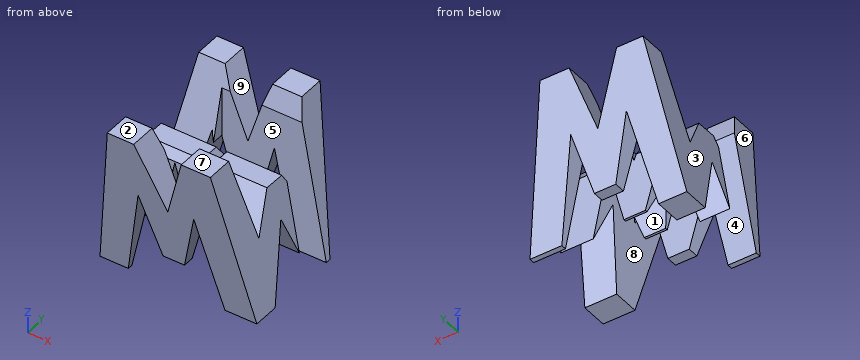
from build123d import *

# Parameters (mm, degrees)
F0_W      = 38.1
F0_H      = 38.1
F1_DEPTH  = 38.1
F6_DEPTH  = 38.1
F8_DEPTH  = 38.1
F9_W      = 25.4
F9_H      = 7.62
F10_DEPTH = 38.1


with BuildPart() as f1:
    # F0 (on Front) → F1 (new body)
    with BuildSketch(Plane.XZ):
        with Locations((19.05, 19.05)):
            Rectangle(F0_W, F0_H)
    extrude(amount=F1_DEPTH)

    # F4 (on face) → F6 (cut)
    with BuildSketch(Plane.YZ.offset(38.1)):
        Polygon((-6.35, 38.1), (-31.75, 38.1), (-26.67, 17.005277), (-21.59, 25.867645), (-16.51, 25.753345), (-11.43, 17.005277), align=None)
        Polygon((-31.75, 0), (-38.1, 38.1), (-38.1, 0), align=None)
        Polygon((0, 0), (0, 38.1), (-6.35, 0), align=None)
        Polygon((-19.05, 17.005277), (-25.4, 0), (-12.7, 0), align=None)
    extrude(amount=-F6_DEPTH, mode=Mode.SUBTRACT)

    # F7 (on offset) → F8 (cut)
    with BuildSketch(Plane.XZ.offset(38.1)):
        Polygon((0, 38.1), (0, 0), (6.205763, 38.1), align=None)
        Polygon((11.968254, 23.367919), (6.870665, 0), (30.363908, 0), (25.482736, 23.367919), (21.498529, 8.313587), (16.292483, 8.313587), align=None)
        Polygon((31.250443, 38.1), (38.1, 0), (38.1, 38.1), align=None)
        Polygon((24.158144, 38.1), (12.633159, 38.1), (19.05, 22.168303), align=None)
    extrude(amount=-F8_DEPTH, mode=Mode.SUBTRACT)

    # F9 (on offset) → F10 (cut)
    with BuildSketch(Plane.XY.offset(38.1)):
        with Locations((25.4, -11.43)):
            Rectangle(F9_W, F9_H)
        with Locations((12.7, -26.67)):
            Rectangle(F9_W, F9_H)
    extrude(amount=-F10_DEPTH, mode=Mode.SUBTRACT)


solid = f1.part
Model file for the job. Use its own axes, mm. Face numbers are marked on the shaded views. A direction names the side the tool comes from. Round coordinates to 2 decimals unless told otherwise and drop trailing zeros. Loops run counter-clockwise (first coordinate to the right, second up) from the corner with the lowest first, then second, coordinate; pieces in that order, holes last. Notation, with made-up numbers: (-40, 26.25) -> (-31, 26.25) arc R34 cw to (-31, 57.25) -> close; hole circle Ø10 at (-6.75, -40). An arc over 180 degrees is marked (long way). Answer as CSV lines item,"result". Start each with the question number.
1) Slice it at B-B (x = 9). List the corners of the cut face in (y, z), plus the area to 3 significant figures.
2) Mould opens along X. For the marked faces 6, 7, 8 and 9 say: +X half, -X half, draft (parallel to the pull), parting line (faces both ways), or undercut.
3) Slice it at C-C (y = -7). List the corners of the cut face in (x, z), plus the area to 3 significant figures.
4) Slice it at A-A (z = 4). List the corners of the cut face in (x, y).
5) Slice it at D-D (z = 31.5). List the corners of the cut face in (x, y).
6) Tool access for the marked faces 1, 2, 3, 4 and 5: list every direction of +Z, -Z, +X, -X, +Y, -Y with a clear straight run to the whole face (end or side of a thin tool).
7) Probe line 1 along Y through (x, z) = (7, 17.5); line 2 along Y through (x, z) = (19, 11.5); line 3 along Y through (x, z) = (7, 14). List the from-to ranges inside material, lowest first.
8) Pin check, flat tips, straight feed: P1, Ø18.5, axis at x = 17, z = 15, coming from the -Y side; P2, Ø0.6, axis at x = 19, y = -15.5, coming from the -Z side; P3, Ø10, axis at x = 11.5, z = 17, coming from the -Y side; P4, Ø1, axis at x = 11.5, z = 18, coming from the +Y side. Stop position of each tip, or through.
Filled in:
1,outline,"(-38.1, 38.1) -> (-33.38, 9.76) -> (-30.48, 9.76) -> (-30.48, 32.83) -> (-31.75, 38.1) -> close; (-22.86, 9.76) -> (-21.76, 9.76) -> (-19.05, 17.01) -> (-16.34, 9.76) -> (-4.72, 9.76) -> (0, 38.1) -> (-6.35, 38.1) -> (-11.43, 17.01) -> (-16.51, 25.75) -> (-21.59, 25.87) -> (-22.86, 23.65) -> close"
1,area,"489 mm2"
2,face 6,"-X half"
2,face 7,"draft"
2,face 8,"undercut"
2,face 9,"undercut"
3,outline,"(0, 0) -> (6.87, 0) -> (11.97, 23.37) -> (16.29, 8.31) -> (21.5, 8.31) -> (25.48, 23.37) -> (30.36, 0) -> (38.1, 0) -> (31.74, 35.4) -> (23.29, 35.4) -> (19.05, 22.17) -> (13.72, 35.4) -> (5.77, 35.4) -> close"
3,area,"779 mm2"
4,outline,"(0.65, -32.42) -> (7.74, -32.42) -> (7.74, -30.48) -> (0.65, -30.48) -> close; (0.65, -14.19) -> (7.74, -14.19) -> (7.74, -5.68) -> (0.65, -5.68) -> close; (29.53, -32.42) -> (37.38, -32.42) -> (37.38, -23.91) -> (29.53, -23.91) -> close; (29.53, -7.62) -> (37.38, -7.62) -> (37.38, -5.68) -> (29.53, -5.68) -> close"
5,outline,"(5.13, -37) -> (15.29, -37) -> (15.29, -30.48) -> (5.13, -30.48) -> close; (5.13, -7.94) -> (12.7, -7.94) -> (12.7, -7.62) -> (15.29, -7.62) -> (15.29, -1.1) -> (5.13, -1.1) -> close; (22.04, -37) -> (32.44, -37) -> (32.44, -30.16) -> (25.4, -30.16) -> (25.4, -30.48) -> (22.04, -30.48) -> close; (22.04, -7.62) -> (32.44, -7.62) -> (32.44, -1.1) -> (22.04, -1.1) -> close"
6,face 1,"-Z, +X, -X"
6,face 2,"+Z, +X, -X, +Y, -Y"
6,face 3,"+Z, -X, +Y, -Y"
6,face 4,"+Z, -Z, -X"
6,face 5,"+Z, -Z, +X"
7,line 1,"y = -34.67 to -30.48, -22.86 to -11.72, -11.31 to -3.43"
7,line 2,"y = -33.67 to -30.48, -22.86 to -21.11, -16.99 to -15.24, -7.62 to -4.43"
7,line 3,"y = -34.08 to -30.48, -22.86 to -20.17, -17.93 to -4.02"
8,P1,"stops at y = -35.79"
8,P2,"stops at z = 8.31"
8,P3,"stops at y = -35.42"
8,P4,"passes through"
